from build123d import *

# Parameters (mm, degrees)
SKETCH_1_R      = 3.25
SKETCH_1_R_2    = 1
EXTRUDE_1_DEPTH = 26


with BuildPart() as part:
    # 草图1 → 凸台-拉伸1 (new, symmetric)
    with BuildSketch(Plane(origin=(0, 0, 0), x_dir=(0, 0, -1), z_dir=(1, 0, 0))):
        with Locations(Location((0, 0, 0), (0, 0, 180))):
            Circle(SKETCH_1_R)
        with Locations(Location((0, 0, 0), (0, 0, 180))):
            Circle(SKETCH_1_R_2, mode=Mode.SUBTRACT)
    extrude(amount=EXTRUDE_1_DEPTH, both=True)

    # 草图2 → 切除-旋转1 (revolve, cut)
    with BuildSketch(Plane.XY, mode=Mode.PRIVATE) as cut_revolve_1_sk:
        Polygon((-17.180633651, 3.25), (18.680633651, 3.25), (16, 2), (-14.5, 2), align=None)
    revolve(cut_revolve_1_sk.sketch.rotate(Axis((-26, 0, 0), (1, 0, 0)), 90), axis=Axis((-26, 0, 0), (1, 0, 0)), mode=Mode.SUBTRACT)


solid = part.part
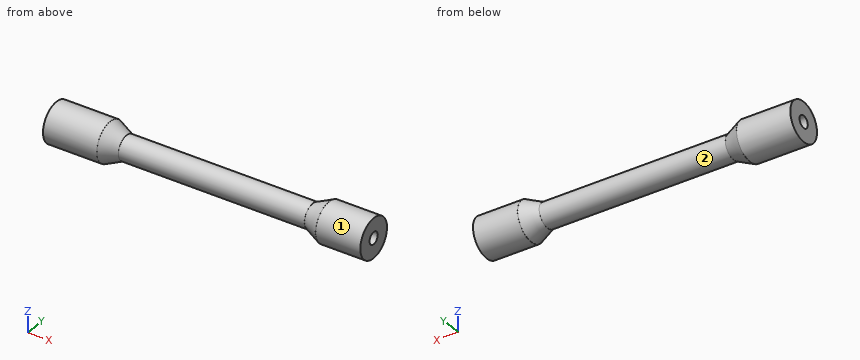
Work out the finished part from the listing and answer in its coordinate system (mm). Face numbers are marked on the shaded views. A direction names the side the tool comes from. Give positions to 0.01 mm unless a question says otherwise; leave off trailing zeros. Order: outer loops, then holes, each group sorted by start corner. A loop starts at its lowest first (then second) coordinate and runs counter-clockwise, first axis right, second up. Notation, with made-up numbers: M 5.25,3 L 39.25,3 A16 cw 39.25,14 Z; hole C -19,67 d9. An arc over 180 degrees is marked long. Return JSON: item names as keys, results as strings.
Q1. Each of these flat-tipped pins is pushed along its axis until it touches: pin 1 (1.2 mm diameter, centred on y = 0, z = 0, fed in from -X); pin 2 (1 mm diameter, centred on x = 0.5, y = 1, fed in from +Z); pin 3 (3 mm diameter, centred on x = 14.5, y = 2, fed in from -Z); pin 4 (1.5 mm diameter, centred on x = -13.5, z = -0.5, fed in from -Y). Where does it stop, or does it pass through?
Answer below:
{"pin 1": "passes through", "pin 2": "stops at z = 1.94", "pin 3": "stops at z = -1.94", "pin 4": "stops at y = -2"}
Q2. Which of the six approach directions +Z, -Z, +X, -X, +Y, -Y give full straight-line access (tool end or side, diameter ignored) to the marked faces 1 and 2?
Answer below:
{"face 1": "+X, -X", "face 2": "none"}
Q3. Find section A-A, the plane z = 0. Write down the section's boundary in (x, y).
Answer below:
{"outline": "M -26,-3.25 L -17.18,-3.25 L -14.5,-2 L 16,-2 L 18.68,-3.25 L 26,-3.25 L 26,-1 L -26,-1 Z; M -26,1 L 26,1 L 26,3.25 L 18.68,3.25 L 16,2 L -14.5,2 L -17.18,3.25 L -26,3.25 Z"}
Q4. Find the intervals of material crossed by line 1 along Y through (x, z) = (-1.5, 0); line 2 along X through (y, z) = (-0.25, -2.5); line 3 along Y through (x, z) = (13, -0.75), in increasing order. Write a range as [from, to].
Answer below:
{"line 1": "y = [-2, -1], [1, 2]", "line 2": "x = [-26, -15.6], [17.1, 26]", "line 3": "y = [-1.85, -0.66], [0.66, 1.85]"}
Q5. Find section C-C, the plane x = 11. Write down the section's boundary in (y, z), and give its area (3 significant figures).
Answer below:
{"outline": "C 0,0 d4; hole C 0,0 d2", "area": "9.42 mm^2"}
Q6. Find section D-D, the plane x = 21. Write down the section's boundary in (y, z).
Answer below:
{"outline": "C 0,0 d6.5; hole C 0,0 d2"}
